For this review, take the finished solid that the model builds, in its own axes (mm). A direction names the side the tool comes from. Coordinates: 2 decimals unless noted, no trailing zeros. Order: outer loops, then holes, each group sorted by start corner. A loop starts at its lowest first (then second) coordinate and runs counter-clockwise, first axis right, second up.
from build123d import *

# Parameters (mm, degrees)
SKETCH1_R                       = 20
SKETCH1_R_2                     = 1
BOSS_EXTRUDE1_DEPTH             = 21.55
TAP_DRILL_FOR_M5X0_8_TAP1_D     = 4.2
TAP_DRILL_FOR_M5X0_8_TAP1_DEPTH = 5
TAP_DRILL_FOR_M5X0_8_TAP1_TIP   = 1.2618073
SKETCH4_W                       = 6.5
SKETCH4_H                       = 6.5
CUT_EXTRUDE1_DEPTH              = 19.05
CIRPATTERN1_COUNT               = 4
SKETCH5_R                       = 6
SKETCH5_R_2                     = 5
SKETCH5_R_3                     = 1
CUT_EXTRUDE2_DEPTH              = 1
CUT_EXTRUDE3_START              = -21.55
SKETCH6_W                       = 10
SKETCH6_H                       = 5.7725
SKETCH6_R                       = 2.1
CUT_EXTRUDE3_DEPTH              = 21.55
SKETCH7_R                       = 10.5
CUT_EXTRUDE4_DEPTH              = 6.55
FILLET4_R                       = 2
FILLET5_R                       = 4


with BuildPart() as part:
    # Sketch1 → Boss-Extrude1 (new body)
    with BuildSketch(Plane.XY):
        with Locations((-11.822558412, 14.529752947)):
            Circle(SKETCH1_R)
        with Locations((-11.822558412, 14.529752947)):
            Circle(SKETCH1_R_2, mode=Mode.SUBTRACT)
    extrude(amount=BOSS_EXTRUDE1_DEPTH)

    # Tap Drill for M5x0.8 Tap1
    with Locations(Plane.XY.offset(21.55)):
        with Locations((-11.822558412, 14.529752947)):
            Hole(TAP_DRILL_FOR_M5X0_8_TAP1_D / 2, depth=TAP_DRILL_FOR_M5X0_8_TAP1_DEPTH)
            with Locations((0, 0, -(TAP_DRILL_FOR_M5X0_8_TAP1_DEPTH + TAP_DRILL_FOR_M5X0_8_TAP1_TIP / 2))):  # 118° drill point
                Cone(0, TAP_DRILL_FOR_M5X0_8_TAP1_D / 2, TAP_DRILL_FOR_M5X0_8_TAP1_TIP, mode=Mode.SUBTRACT)

    # Sketch4 → Cut-Extrude1 (cut)
    with BuildSketch(Plane.XY.offset(21.55)):
        with Locations((2.927441588, 14.529752947)):
            Rectangle(SKETCH4_W, SKETCH4_H)
    cut_extrude1 = extrude(amount=-CUT_EXTRUDE1_DEPTH, mode=Mode.SUBTRACT)

    # CirPattern1: Cut-Extrude1 ×4 about axis
    cirpattern1_axis = Axis((-11.822558412, 14.529752947, 0), (0, 0, 1))
    for i in range(1, CIRPATTERN1_COUNT):
        add(cut_extrude1.rotate(cirpattern1_axis, i * 360 / CIRPATTERN1_COUNT), mode=Mode.SUBTRACT)

    # Sketch5 → Cut-Extrude2 (cut)
    # profile 1 of 2: a face of its own
    with BuildSketch(Plane(origin=(0, 0, 0), x_dir=(-1, 0, 0), z_dir=(0, 0, -1))):
        with Locations((11.822558412, 14.529752947)):
            Circle(SKETCH5_R)
        with Locations((11.822558412, 14.529752947)):
            Circle(SKETCH5_R_2, mode=Mode.SUBTRACT)
    # profile 2 of 2: a face of its own
    with BuildSketch(Plane(origin=(0, 0, 0), x_dir=(-1, 0, 0), z_dir=(0, 0, -1))):
        with Locations((11.822558412, 14.529752947)):
            Circle(SKETCH5_R_2)
        with Locations((11.822558412, 14.529752947)):
            Circle(SKETCH5_R_3, mode=Mode.SUBTRACT)
    extrude(amount=-CUT_EXTRUDE2_DEPTH, mode=Mode.SUBTRACT)

    # Sketch6 → Cut-Extrude3 (cut)
    # profile 1 of 4: a face of its own
    with BuildSketch(Plane.XY.offset(21.55).offset(CUT_EXTRUDE3_START)):
        with Locations((-11.822558412, 14.529752947)):
            Rectangle(SKETCH6_W, SKETCH6_H)
        with Locations((-11.822558412, 14.529752947)):
            Circle(SKETCH6_R, mode=Mode.SUBTRACT)
    # profile 2 of 4: a face of its own
    with BuildSketch(Plane.XY.offset(21.55).offset(CUT_EXTRUDE3_START)):
        with Locations((-11.822558412, 14.529752947)):
            Circle(SKETCH6_R)
    # profile 3 of 4: a face of its own
    with BuildSketch(Plane.XY.offset(21.55).offset(CUT_EXTRUDE3_START)):
        Polygon((-11.822558412, 20.295742519), (-6.822558412, 17.416002947), (-16.822558412, 17.416002947), align=None)
    # profile 4 of 4: a face of its own
    with BuildSketch(Plane.XY.offset(21.55).offset(CUT_EXTRUDE3_START)):
        Polygon((-11.822558412, 8.763763375), (-16.822558412, 11.643502947), (-6.822558412, 11.643502947), align=None)
    extrude(amount=CUT_EXTRUDE3_DEPTH, mode=Mode.SUBTRACT)

    # Sketch7 → Cut-Extrude4 (cut)
    with BuildSketch(Plane.XY.offset(21.55)):
        with Locations((-11.822558412, 14.529752947)):
            Circle(SKETCH7_R)
    extrude(amount=-CUT_EXTRUDE4_DEPTH, mode=Mode.SUBTRACT)

    # Fillet4
    # the kernel refuses this fillet: 2 mm, written as the material it takes off along each edge
    with BuildSketch(Plane(origin=(-11.822558412, 14.529752947, 21.55), x_dir=(1, 0, 0), z_dir=(0, -1, 0))) as fillet4_piece_1:
        with BuildLine():
            CenterArc((10.5 + FILLET4_R, -FILLET4_R), FILLET4_R, 90, 90)
            Line((10.5, -FILLET4_R), (10.5, 0))
            Line((10.5, 0), (10.5 + FILLET4_R, 0))
        make_face()
    revolve(axis=Axis((-11.822558412, 14.529752947, 21.55), (0, 0, 1)), mode=Mode.SUBTRACT)

    # Fillet5
    fillet5_edges = [part.edges().sort_by_distance(p)[0] for p in [
        (-22.322558412, 14.529752947, 15),
    ]]
    fillet(fillet5_edges, radius=FILLET5_R)


solid = part.part
1. Take a section at A-A, the plane z = 16. Give the boundary of the cut face in (x, y), plus the area to 3 significant figures.
Answer below:
outline: circle Ø40 at (-11.82, 14.53); hole (-29.82, 11.28) - (-23.32, 11.28) - (-23.32, 17.78) - (-29.82, 17.78) - close; hole circle Ø18.29 at (-11.82, 14.53); hole (-15.07, -3.47) - (-8.57, -3.47) - (-8.57, 3.03) - (-15.07, 3.03) - close; hole (-15.07, 26.03) - (-8.57, 26.03) - (-8.57, 32.53) - (-15.07, 32.53) - close; hole (-0.32, 11.28) - (6.18, 11.28) - (6.18, 17.78) - (-0.32, 17.78) - close
area: 825 mm2
2. Machinability: for faces 4 (the face through (-12, 0, 2.5)), 5 (the face through (-10.522, 8.672, 0.493)), 6 (the face through (-6.823, 14, 8)), which of the approach directions +Z, -Z, +X, -X, +Y, -Y give a long, thin tool a straight path to every point of the face, cutting with its end or side? Answer none if there is none.
Answer below:
face 4: +Z
face 5: -Z
face 6: +Z, -Z
3. To check wall thickness, follow L1, parallel to Y at x = -14.5, z = 17.25; L2, parallel to Y at x = -10, z = 3.75; L3, parallel to X at y = 13, z = 6.75. State the ranges of each line that lie inside material, in increasing order.
Answer below:
L1: y = -5.29 to -3.47, 3.03 to 4.79, 24.27 to 26.03, 32.53 to 34.35
L2: y = -5.39 to -3.47, 3.03 to 9.81, 19.25 to 26.03, 32.53 to 34.45
L3: x = -31.76 to -29.82, -23.32 to -16.82, -6.82 to -0.32, 6.18 to 8.12
4. Clearance check with flat-ended pins moving along their axes: pin 1 Ø10 at (x, z) = (-9, 5.5) entering from +Y; pin 2 Ø3 at (x, y) = (-11, 1) entering from +Z; pin 3 Ø10 at (x, z) = (-23.5, 9) entering from -Y. State where each tip first meets the part, or that it passes through.
Answer below:
pin 1: stops at y = 34.53
pin 2: stops at z = 2.5
pin 3: stops at y = -4.32
5. The part is to be moulded in two halves that separate along X. For faces 1 (the face through (-23.323, 15, 12)), 2 (the face through (-3, 24, 21.55)), 3 (the face through (-27.694, 2.36, 10.624)), say which applies: +X half, -X half, draft (parallel to the pull), parting line (faces both ways), or undercut.
Answer below:
face 1: undercut
face 2: draft
face 3: parting line
6. Take a section at B-B, the plane y = -2. Give the boundary of the cut face in (x, z), plus the area to 3 significant figures.
Answer below:
outline: (-23.08, 0) - (-0.56, 0) - (-0.56, 21.55) - (-8.57, 21.55) - (-8.57, 2.5) - (-15.07, 2.5) - (-15.07, 21.55) - (-23.08, 21.55) - close
area: 361 mm2
7. Take a section at C-C, the plane x = 1.5. Give the boundary of the cut face in (y, z), plus the area to 3 significant figures.
Answer below:
outline: (-0.39, 0) - (29.45, 0) - (29.45, 21.55) - (17.78, 21.55) - (17.78, 2.5) - (11.28, 2.5) - (11.28, 21.55) - (-0.39, 21.55) - close
area: 519 mm2
8. Take a section at D-D, the plane z = 3.5. Give the boundary of the cut face in (x, y), plus the area to 3 significant figures.
Answer below:
outline: circle Ø40 at (-11.82, 14.53); hole (-29.82, 11.28) - (-23.32, 11.28) - (-23.32, 17.78) - (-29.82, 17.78) - close; hole (-16.82, 11.64) - (-11.82, 8.76) - (-6.82, 11.64) - (-6.82, 17.42) - (-11.82, 20.3) - (-16.82, 17.42) - close; hole (-15.07, -3.47) - (-8.57, -3.47) - (-8.57, 3.03) - (-15.07, 3.03) - close; hole (-15.07, 26.03) - (-8.57, 26.03) - (-8.57, 32.53) - (-15.07, 32.53) - close; hole (-0.32, 11.28) - (6.18, 11.28) - (6.18, 17.78) - (-0.32, 17.78) - close
area: 1,000 mm2
